Verification items for the finished model (mm, model axes). Face numbers are marked on the shaded views. A direction names the side the tool comes from. Give positions to 0.01 mm unless a question says otherwise; leave off trailing zeros. Order: outer loops, then holes, each group sorted by start corner. A loop starts at its lowest first (then second) coordinate and runs counter-clockwise, first axis right, second up.
from build123d import *

# Parameters (mm, degrees)
SKETCH1_R           = 1.7499999999999998
SKETCH1_R_2         = 1.7500000000000002
BOSS_EXTRUDE1_DEPTH = 8.5
BOSS_EXTRUDE2_START = -8.5
BOSS_EXTRUDE2_DEPTH = 8.5
FILLET1_R           = 2


with BuildPart() as part:
    # Sketch1 → Boss-Extrude1 (new body)
    with BuildSketch(Plane(origin=(0, 0, 0), x_dir=(0, 0, -1), z_dir=(1, 0, 0))):
        with BuildLine():
            Line((27, 10), (4.999999999999845, 10))
            ThreePointArc((4.999999999999845, 9.999999999999996), (2.66e-15, 4.999999999999989), (4.999999999999866, 2.66e-15))
            Line((4.999999999999866, 0), (27, 0))
            ThreePointArc((27, -8.9e-16), (32, 5), (27, 10))
        make_face()
        with Locations((5, 5)):
            Circle(SKETCH1_R, mode=Mode.SUBTRACT)
        with Locations((27, 5)):
            Circle(SKETCH1_R_2, mode=Mode.SUBTRACT)
    extrude(amount=BOSS_EXTRUDE1_DEPTH)

    # Sketch2 → Boss-Extrude2 (add)
    with BuildSketch(Plane(origin=(8.5, 0, 0), x_dir=(0, 0, -1), z_dir=(1, 0, 0)).offset(BOSS_EXTRUDE2_START)):
        with BuildLine():
            add(Edge.make_bspline(
                [(63.753003749139694, 17.8724364513696), (48.4484123726985, 16.075931173157382), (33.927648133343, 10.00000000000011), (18.35740593050513, 10)],
                knots=[0, 0, 0, 0, 1, 1, 1, 1], degree=3))
            Line((18.35740593050513, 10), (27, 10.000000000000002))
            ThreePointArc((27, 10.000000000000004), (31.76198872224619, 6.524291116945876), (29.90346284332652, 0.9293853636800407))
            Line((29.903462843326523, 0.9293853636800362), (37.27788733358429, 6.189369275529155))
            add(Edge.make_bspline(
                [(37.27788733358429, 6.189369275529155), (48.425576395597574, 11.344056029156562), (60.710162222104955, 12.2385110488325)],
                knots=[0, 0, 0, 1, 1, 1], degree=2))
            Line((60.710162222104955, 12.238511048832498), (65.58908690842728, 13.539967250903384))
            Line((65.58908690842728, 13.539967250903384), (63.753003749139694, 17.8724364513696))
        make_face()
    extrude(amount=BOSS_EXTRUDE2_DEPTH)

    # Sketch3 → Cut-Revolve1 (revolve, cut)
    with BuildSketch(Plane.ZY.offset(-4.25)):
        with BuildLine():
            Line((-61.363286830934264, 3.0092373204057665), (-70.57054843387056, 6.911330832239489))
            add(Edge.make_bspline(
                [(-61.363286830934264, 3.0092373204057665), (-56.87587929232551, 13.597588163782518), (-61.47951009379365, 15.548634919699378), (-66.08314089526179, 17.499681675616234), (-70.57054843387056, 6.911330832239489)],
                knots=[1.5707963267948968, 1.5707963267948968, 1.5707963267948968, 3.141592653589793, 3.141592653589793, 4.71238898038469, 4.71238898038469, 4.71238898038469], degree=2, weights=[1, 0.7071067811865477, 1, 0.7071067811865477, 1]))
        make_face()
    revolve(axis=Axis((4.25, 3.0092373204057665, -61.363286830934264), (0, 0.3902093511833724, -0.9207261602936302)), mode=Mode.SUBTRACT)

    # Fillet1
    fillet1_edges = [part.edges().sort_by_distance(p)[0] for p in [
        (4.25, 17.8724364513696, -63.753003749139694),
    ]]
    fillet(fillet1_edges, radius=FILLET1_R)

    # Sketch4 → Cut-Revolve4 (revolve, cut)
    with BuildSketch(Plane(origin=(0, 24.455596913653128, -57.70468538416743), x_dir=(0, -0.9207261602936302, -0.39020935118337224), z_dir=(0, 0.39020935118337224, -0.9207261602936302))):
        with BuildLine():
            Line((21.173844817348538, 0.7500000000000007), (21.173844817348538, -9.250000000000004))
            add(Edge.make_bspline(
                [(21.173844817348538, 0.7500000000000007), (9.67384481734854, 0.7500000000000027), (9.673844817348536, -4.249999999999997), (9.673844817348535, -9.249999999999996), (21.173844817348538, -9.250000000000004)],
                knots=[4.71238898038469, 4.71238898038469, 4.71238898038469, 6.283185307179586, 6.283185307179586, 7.853981633974483, 7.853981633974483, 7.853981633974483], degree=2, weights=[1, 0.7071067811865476, 1, 0.7071067811865476, 1]))
        make_face()
    revolve(axis=Axis((-0.7500000000000007, 4.960284076322628, -65.96691763240241), (1, 0, 0)), mode=Mode.SUBTRACT)


solid = part.part
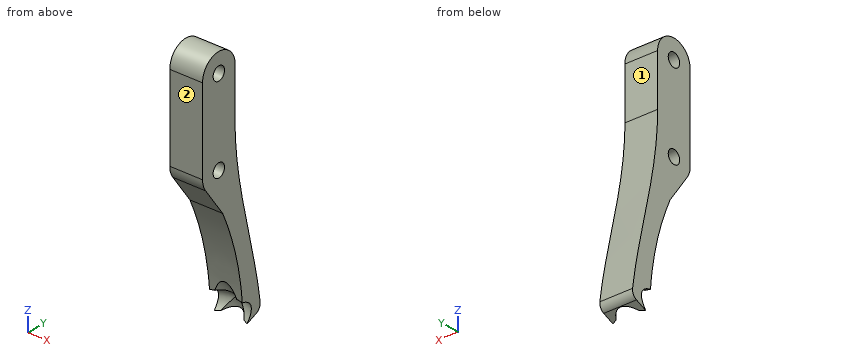
(1) Section check D-D, the plane y = 2.5. Enter the section's corners in (x, z), then the cut area to 3 significant figures.
Solved:
outline: (0, -32.11) - (8.5, -32.11) - (8.5, -0.67) - (0, -0.67) - close
area: 267 mm2
(2) Section check C-C, the plane x = 3. Give the number of separate pieces and of enclosed holes in the cut face, then the cut area to 4 significant figures.
Solved:
separate pieces: 1
enclosed holes: 2
area: 452.5 mm2
(3) Section check A-A, the plane y = 5. Enter the section's corners in (x, z).
Solved:
outline: (0, -35.61) - (8.5, -35.61) - (8.5, -28.75) - (0, -28.75) - close; (0, -25.25) - (8.5, -25.25) - (8.5, -6.75) - (0, -6.75) - close; (0, -3.25) - (8.5, -3.25) - (8.5, 0) - (0, 0) - close
(4) Set-up check for the marked faces 1 and 2: record each of +Z, -Z, +X, -X, +Y, -Y from which the full face is reachable in a straight line by a thin tool's end or side.
Solved:
face 1: +Z, +X, -X, +Y
face 2: +Z, -Z, +X, -X, -Y
(5) Section check B-B, the plane z = -17. Enter the section's corners in (x, y).
Solved:
outline: (0, 0) - (8.5, 0) - (8.5, 10) - (0, 10) - close
(6) Go/stop test with flat-tipped pins: pin 1 (1 mm diameter, centred on y = 11.5, z = -32, fed in from -X); pin 2 (4 mm diameter, centred on x = 2.5, z = -10, fed in from +Y); pin 3 (4 mm diameter, centred on x = 3.5, z = -55.5, fed in from -Y); pin 4 (3 mm diameter, centred on x = 2, z = -31.5, fed in from -Y). Record where each tip stops, or that it passes through.
Solved:
pin 1: stops at x = 0
pin 2: stops at y = 10
pin 3: stops at y = 11.33
pin 4: stops at y = 1
(7) Scan lines: line 1 (Y direction, x = 6, z = -27); line 2 (Y direction, x = 7.5, z = -15.5); line 3 (Y direction, x = 2, z = -36). Record each from-to range of solid material in increasing order.
Solved:
line 1: y = 0 to 3.25, 6.75 to 10.57
line 2: y = 0 to 10
line 3: y = 5.28 to 12.12
